Autodesk Inventor part; units mm, degrees
ref_plane "YZ Plane" through (0, 0, 0) normal (1, 0, 0) x (0, 1, 0)
ref_plane "XZ Plane" through (0, 0, 0) normal (0, 1, 0) x (-1, 0, 0)
ref_plane "XY Plane" through (0, 0, 0) normal (0, 0, 1) x (1, 0, 0)
sketch "Sketch1" plane through (0, 0, 0) normal (0, 0, 1) x (1, 0, 0)
  line L0 (0, 0) -> (0, 25.4)
  line L1 (0, 25.4) -> (101.6, 25.4)
  line L2 (101.6, 25.4) -> (101.6, 0)
  line L3 (101.6, 0) -> (0, 0)
  circle A0 centre (22.225, 12.7) radius 3.3782
  circle A1 centre (88.9, 12.7) radius 3.3782
  circle A2 centre (53.975, 12.7) radius 3.3782
  dimension "d0" = 25.4
  dimension "d1" = 101.6
  dimension "d2" = 6.7564
  dimension "d3" = 6.7564
  dimension "d4" = 22.225
  dimension "d5" = 12.7
  dimension "d6" = 12.7
  dimension "d7" = 12.7
  dimension "d10" = 6.7564
  dimension "d11" = 31.75
  dimension "d14" = 12.7
extrude "Extrusion2" add sketch "Sketch1" along normal blind 3.175
properties part number "Gusset 3" material "Aluminum 6061"
Geometry check sheet. Reference: the model listing, model coordinates, mm. Coordinates: 2 decimals unless noted, no trailing zeros. Loops run counter-clockwise (first coordinate to the right, second up) from the corner with the lowest first, then second, coordinate; pieces in that order, holes last.
Item 1: Sectioned sample at B-B, the plane x = 88.9. Record the boundary of the cut face in (y, z) (3 decimals).
Item 2: Sectioned sample at A-A, the plane y = 12.7. Record the boundary of the cut face in (x, z) (3 decimals), then the cut area to 3 significant figures.
Item 3: Thickness scan on line 1 (Y direction, x = 54, z = 2.75); line 2 (X direction, y = 12.25, z = 2.45); line 3 (X direction, y = 13.75, z = 1.65). Record the ranges inside material, lowest first.
Item 4: Release check for a two-part mould opening along X. For faces 1 (the face through (19.544, 14.756, 1.565)), 2 (the face through (0, 13, 2)), 3 (the face through (53.243, 15.998, 1.565)), 4 (the face through (50, 13, 0)) record: released by +X, released by -X, zero draft, split by the parting line, or undercut.
Item 5: Go/stop test with flat-tipped pins: pin 1 Ø5.5 at (x, y) = (53.975, 12.7) entering from -Z; pin 2 Ø2 at (x, y) = (71.5, 7.5) entering from -Z. Record where each tip stops, or that it passes through.
Item 6: Sectioned sample at C-C, the plane z = 0.6. Record the boundary of the cut face in (x, y) (3 decimals), then the cut area to 3 significant figures.
Check result:
1. outline: (0, 0) - (9.322, 0) - (9.322, 3.175) - (0, 3.175) - close; (16.078, 0) - (25.4, 0) - (25.4, 3.175) - (16.078, 3.175) - close
2. outline: (0, 0) - (18.847, 0) - (18.847, 3.175) - (0, 3.175) - close; (25.603, 0) - (50.597, 0) - (50.597, 3.175) - (25.603, 3.175) - close; (57.353, 0) - (85.522, 0) - (85.522, 3.175) - (57.353, 3.175) - close; (92.278, 0) - (101.6, 0) - (101.6, 3.175) - (92.278, 3.175) - close
2. area: 258 mm2
3. line 1: y = 0 to 9.32, 16.08 to 25.4
3. line 2: x = 0 to 18.88, 25.57 to 50.63, 57.32 to 85.55, 92.25 to 101.6
3. line 3: x = 0 to 19.01, 25.44 to 50.76, 57.19 to 85.69, 92.11 to 101.6
4. face 1: undercut
4. face 2: released by -X
4. face 3: undercut
4. face 4: zero draft
5. pin 1: passes through
5. pin 2: stops at z = 0
6. outline: (0, 0) - (101.6, 0) - (101.6, 25.4) - (0, 25.4) - close; hole circle Ø6.756 at (22.225, 12.7); hole circle Ø6.756 at (53.975, 12.7); hole circle Ø6.756 at (88.9, 12.7)
6. area: 2,470 mm2
